from build123d import *

# Parameters (mm, degrees)
BOSS_EXTRUDE1_DEPTH = 114.3
SKETCH8_R           = 1.778
CUT_EXTRUDE1_DEPTH  = 5.08
SKETCH9_R           = 1.778
CUT_EXTRUDE2_DEPTH  = 5.08
SKETCH10_R          = 1.778
CUT_EXTRUDE3_DEPTH  = 5.08
SKETCH13_R          = 1.778
CUT_EXTRUDE6_DEPTH  = 5.08
CUT_EXTRUDE7_DEPTH  = 2.54
SKETCH16_W          = 19.05
SKETCH16_H          = 1.27
CUT_EXTRUDE8_DEPTH  = 47.625
SKETCH17_W          = 8.89
SKETCH17_H          = 8.89
CUT_EXTRUDE9_DEPTH  = 38.1
SKETCH18_W          = 8.89
SKETCH18_H          = 8.89
CUT_EXTRUDE10_DEPTH = 2.54


with BuildPart() as part:
    # Sketch1 → Boss-Extrude1 (new body)
    with BuildSketch(Plane(origin=(0, 0, 0), x_dir=(1, 0, 0), z_dir=(0, 1, 0))):
        Polygon((23.749, 23.749), (-23.749, 23.749), (-23.749, -23.749), (-22.479, -23.749), (-22.479, 22.479), (22.479, 22.479), (22.479, -23.749), (23.749, -23.749), align=None)
    extrude(amount=BOSS_EXTRUDE1_DEPTH)

    # Sketch8 → Cut-Extrude1 (cut)
    with BuildSketch(Plane(origin=(0, 0, -23.749), x_dir=(-1, 0, 0), z_dir=(0, 0, -1))):
        with Locations((0, 57.15)):
            Circle(SKETCH8_R)
    extrude(amount=-CUT_EXTRUDE1_DEPTH, mode=Mode.SUBTRACT)

    # Sketch9 → Cut-Extrude2 (cut)
    with BuildSketch(Plane.ZY.offset(23.749)):
        with Locations((0, 38.1)):
            Circle(SKETCH9_R)
    extrude(amount=-CUT_EXTRUDE2_DEPTH, mode=Mode.SUBTRACT)

    # Sketch10 → Cut-Extrude3 (cut)
    with BuildSketch(Plane(origin=(23.749, 0, 0), x_dir=(0, 0, -1), z_dir=(1, 0, 0))):
        with Locations((0, 88.9)):
            Circle(SKETCH10_R)
    extrude(amount=-CUT_EXTRUDE3_DEPTH, mode=Mode.SUBTRACT)

    # Sketch13 → Cut-Extrude6 (cut)
    with BuildSketch(Plane(origin=(0, 0, -23.749), x_dir=(-1, 0, 0), z_dir=(0, 0, -1))):
        with Locations((0, 25.4)):
            Circle(SKETCH13_R)
    extrude(amount=-CUT_EXTRUDE6_DEPTH, mode=Mode.SUBTRACT)

    # Sketch14 → Cut-Extrude7 (cut)
    with BuildSketch(Plane.ZY.offset(23.749)):
        with BuildLine():
            Line((-17.018, 99.6), (-17.018, 101.6))
            Line((-17.018, 101.6), (-15.018, 101.6))
            ThreePointArc((-15.018, 101.6), (-18.432213562, 103.014213562), (-17.018, 99.6))
        make_face()
        with BuildLine():
            Line((-15.018, 101.6), (-17.018, 101.6))
            Line((-17.018, 101.6), (-17.018, 99.6))
            ThreePointArc((-17.018, 99.6), (-15.603786438, 100.185786438), (-15.018, 101.6))
        make_face()
        with BuildLine():
            ThreePointArc((15.482, 101.6), (13.482, 103.6), (11.482, 101.6))
            Line((11.482, 101.6), (13.482, 101.6))
            Line((13.482, 101.6), (13.482, 99.6))
            ThreePointArc((13.482, 99.6), (14.896213562, 100.185786438), (15.482, 101.6))
        make_face()
        with BuildLine():
            Line((13.482, 101.6), (11.482, 101.6))
            ThreePointArc((11.482, 101.6), (12.067786438, 100.185786438), (13.482, 99.6))
            Line((13.482, 99.6), (13.482, 101.6))
        make_face()
        with BuildLine():
            ThreePointArc((15.482, 71.1), (14.896213562, 72.514213562), (13.482, 73.1))
            Line((13.482, 73.1), (13.482, 71.1))
            Line((13.482, 71.1), (11.482, 71.1))
            ThreePointArc((11.482, 71.1), (13.482, 69.1), (15.482, 71.1))
        make_face()
        with BuildLine():
            Line((13.482, 71.1), (13.482, 73.1))
            ThreePointArc((13.482, 73.1), (12.067786438, 72.514213562), (11.482, 71.1))
            Line((11.482, 71.1), (13.482, 71.1))
        make_face()
        with BuildLine():
            ThreePointArc((-15.018, 71.1), (-15.603786438, 72.514213562), (-17.018, 73.1))
            Line((-17.018, 73.1), (-17.018, 71.1))
            Line((-17.018, 71.1), (-15.018, 71.1))
        make_face()
        with BuildLine():
            Line((-17.018, 71.1), (-17.018, 73.1))
            ThreePointArc((-17.018, 73.1), (-18.432213562, 69.685786438), (-15.018, 71.1))
            Line((-15.018, 71.1), (-17.018, 71.1))
        make_face()
    extrude(amount=-CUT_EXTRUDE7_DEPTH, mode=Mode.SUBTRACT)

    # Sketch16 → Cut-Extrude8 (cut)
    with BuildSketch(Plane(origin=(0, 114.3, 0), x_dir=(1, 0, 0), z_dir=(0, 1, 0))):
        with Locations((-14.224, 23.114)):
            Rectangle(SKETCH16_W, SKETCH16_H)
    extrude(amount=-CUT_EXTRUDE8_DEPTH, mode=Mode.SUBTRACT)

    # Sketch17 → Cut-Extrude9 (cut)
    with BuildSketch(Plane.ZY.offset(23.749)):
        with Locations((19.304, 109.855)):
            Rectangle(SKETCH17_W, SKETCH17_H)
    extrude(amount=-CUT_EXTRUDE9_DEPTH, mode=Mode.SUBTRACT)

    # Sketch18 → Cut-Extrude10 (cut)
    with BuildSketch(Plane(origin=(23.749, 0, 0), x_dir=(0, 0, -1), z_dir=(1, 0, 0))):
        with Locations((19.304, 109.855)):
            Rectangle(SKETCH18_W, SKETCH18_H)
    extrude(amount=-CUT_EXTRUDE10_DEPTH, mode=Mode.SUBTRACT)


solid = part.part
Can you work these out from the model? Positions are in its coordinate system, mm. A direction names the side the tool comes from. Give positions to 0.01 mm unless a question says otherwise; leave off trailing zeros. Loops run counter-clockwise (first coordinate to the right, second up) from the corner with the lowest first, then second, coordinate; pieces in that order, holes last. Notation, with made-up numbers: (45, 3) - (50, 3) arc R24 ccw to (50, 41) - close; hole circle Ø2 at (79, 80). An arc over 180 degrees is marked (long way). Return JSON: item names as keys, results as strings.
1. I want a section at A-A on y = 25.4. Please give me the cut outline in (x, z).
Output values:
{"outline": "(-23.75, -23.75) - (-1.78, -23.75) - (-1.78, -22.48) - (-22.48, -22.48) - (-22.48, 23.75) - (-23.75, 23.75) - close; (1.78, -23.75) - (23.75, -23.75) - (23.75, 23.75) - (22.48, 23.75) - (22.48, -22.48) - (1.78, -22.48) - close"}
2. I want a section at B-B on x = 0. Please give me the cut outline in (y, z).
Output values:
{"outline": "(0, -23.75) - (23.62, -23.75) - (23.62, -22.48) - (0, -22.48) - close; (27.18, -23.75) - (55.37, -23.75) - (55.37, -22.48) - (27.18, -22.48) - close; (58.93, -23.75) - (114.3, -23.75) - (114.3, -22.48) - (58.93, -22.48) - close"}
3. We'd pull the mould along X, two halves only. Please class faces 4 (the face through (-23.749, 56, 0)), 5 (the face through (23.749, 56, 0)), 6 (the face through (5, 44, -22.479)), 7 (the face through (23, 105.41, -19)): +X half, -X half, draft (parallel to the pull), parting line (faces both ways), or undercut.
Output values:
{"face 4": "-X half", "face 5": "+X half", "face 6": "undercut", "face 7": "draft"}
4. I want a section at D-D on y = 92. Please give me the cut outline in (x, z).
Output values:
{"outline": "(-23.75, -22.48) - (-22.48, -22.48) - (-22.48, 23.75) - (-23.75, 23.75) - close; (-4.7, -23.75) - (23.75, -23.75) - (23.75, 23.75) - (22.48, 23.75) - (22.48, -22.48) - (-4.7, -22.48) - close"}
5. I'm going to push flat-ended pins straight in: pin 1 Ø1 at (x, y) = (-23, 111.5) entering from +Z; pin 2 Ø1 at (y, z) = (111, -23) entering from +X; pin 3 Ø22.5 at (x, y) = (7.5, 43.5) entering from +Z. Where does each tip first touch, or does it pass through?
Output values:
{"pin 1": "stops at z = 14.86", "pin 2": "stops at x = 21.21", "pin 3": "stops at z = -22.48"}
6. If I drill on line 1 (Z direction, x = -23.35, y = 101.6); line 2 (Y direction, x = 0, z = -23.4); line 3 (Y direction, x = -23.15, z = 0), over which ranges is the centre line in solid material (lowest first)?
Output values:
{"line 1": "z = -22.48 to -19.02, -15.02 to 11.48, 15.48 to 23.75", "line 2": "y = 0 to 23.62, 27.18 to 55.37, 58.93 to 114.3", "line 3": "y = 0 to 36.32, 39.88 to 114.3"}
7. For faces 1 (the face through (-22.479, 56, 1)), 2 (the face through (23.12, 87.82, 1.41)), 3 (the face through (-23.12, 39.3, -1.31)), which set-ups out of +Z, -Z, +X, -X, +Y, -Y let a thin tool reach every point of the face, with its end or its side?
Output values:
{"face 1": "+Z, +Y, -Y", "face 2": "+X", "face 3": "-X"}
8. I want a section at C-C on z = -9.5. Please give me the cut outline in (x, y).
Output values:
{"outline": "(-23.75, 0) - (-22.48, 0) - (-22.48, 114.3) - (-23.75, 114.3) - close; (22.48, 0) - (23.75, 0) - (23.75, 114.3) - (22.48, 114.3) - close"}
